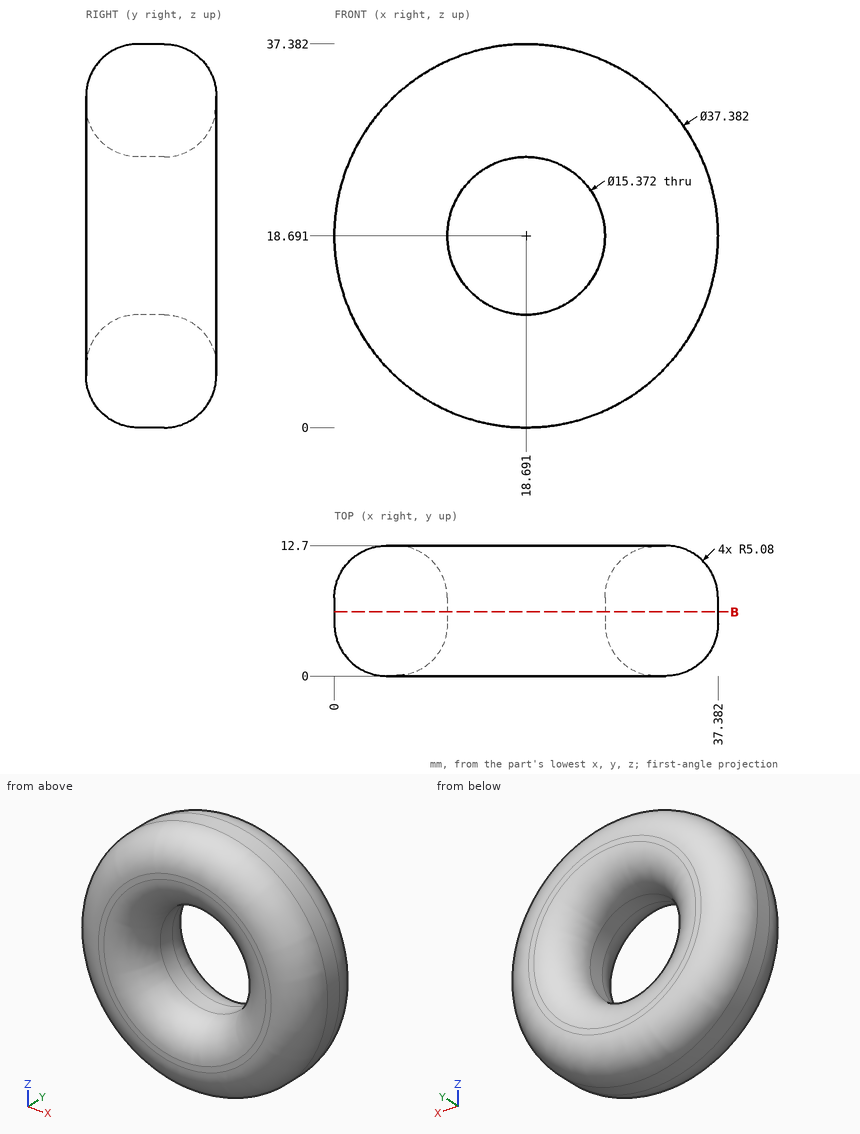
Source: three-view drawing plus pictorial views. Frame: mm from the lowest corner of the part. Round coordinates to 2 decimals unless told otherwise and drop trailing zeros. Order: outer loops, then holes, each group sorted by start corner. A loop starts at its lowest first (then second) coordinate and runs counter-clockwise, first axis right, second up. Notation, with made-up numbers: (-5, -2.5) -> (46, -2.5) arc R24 cw to (46, 36.5) -> close; hole circle Ø4 at (53.5, 6.5). An arc over 180 degrees is marked (long way). Use one line per item in the form item = value.
(1) Section B-B on y = 6.25. Return loops of the section in (x, z), and give its area (3 significant figures).
Results list:
outline = circle Ø37.38 at (18.69, 18.69); hole circle Ø15.37 at (18.69, 18.69)
area = 912 mm^2
(2) First-contact query: pin 1 Ø1.5 at (x, z) = (24.5, 13.5) entering from -Y; pin 2 Ø3 at (x, y) = (12, 3) entering from +Z; pin 3 Ø1.5 at (x, z) = (8.5, 26) entering from -Y; pin 4 Ø2 at (x, y) = (13.5, 2) entering from -Z. Flat tips, straight axial feed; report the tip coordinate or a pass-through.
Results list:
pin_1 = 2.26
pin_2 = 36.41
pin_3 = 0
pin_4 = 1.12
(3) Ray query, probe 1 along X at (y, z) = (5.5, 21); probe 2 along Z at (x, y) = (26.5, 1.75) (1 decimal); probe 3 along X at (y, z) = (9.75, 23) (1 decimal). Return the intervals inside material, ascending. Write a range as [from, to].
Results list:
probe_1 = [0.14, 11.36], [26.02, 37.24]
probe_2 = [3.1, 14.4], [23, 34.3]
probe_3 = [1, 11.8], [25.6, 36.4]
